Autodesk Inventor part; units mm, degrees
ref_plane "YZ Plane" through (0, 0, 0) normal (1, 0, 0) x (0, 1, 0)
ref_plane "XZ Plane" through (0, 0, 0) normal (0, 1, 0) x (-1, 0, 0)
ref_plane "XY Plane" through (0, 0, 0) normal (0, 0, 1) x (1, 0, 0)
sketch "Sketch1" plane through (0, 0, 0) normal (0, 1, 0) x (-1, 0, 0)
  line L0 (0, 0) -> (-21, 0) construction
  line L1 (-4.5, 4.5) -> (-16.5, 4.5)
  line L2 (-16.5, -4.5) -> (-4.5, -4.5)
  arc A0 (-4.5, -4.5) -> (-4.5, 4.5) centre (-4.5, 0) ccw
  arc A1 (-16.5, 4.5) -> (-16.5, -4.5) centre (-16.5, 0) ccw
  point P0 (-10.5, 0)
  dimension "d0" = 9
  dimension "d1" = 21
extrude "Extrusion1" add sketch "Sketch1" along normal blind 4
hole "Hole1" at (4.5, 4, 0) direction (0, -1, 0) diameter 4 end through all
hole "Hole2" at (16.5, 4, 0) direction (0, -1, 0) diameter 4 end through all
properties part number "A8-0015"
Verification items for the finished model (mm, model axes). Round coordinates to 2 decimals unless told otherwise and drop trailing zeros. Loops run counter-clockwise (first coordinate to the right, second up) from the corner with the lowest first, then second, coordinate; pieces in that order, holes last. Notation, with made-up numbers: (80.5, 73) - (89.5, 73) arc R14 cw to (89.5, 90) - close; hole circle Ø9 at (85.25, 33). An arc over 180 degrees is marked (long way). Use one line per item in the form item = value.
1. Section check D-D on z = -3.5. Record the cut outline in (x, y).
A:
outline = (1.67, 0) - (19.33, 0) - (19.33, 4) - (1.67, 4) - close
2. Scan lines: probe 1 along X at (y, z) = (1.15, 0); probe 2 along Z at (x, y) = (16.5, 1.9); probe 3 along Z at (x, y) = (18, 0.6). Record each from-to range of solid material in increasing order.
A:
probe_1 = 0 to 2.5, 6.5 to 14.5, 18.5 to 21
probe_2 = -4.5 to -2, 2 to 4.5
probe_3 = -4.24 to -1.32, 1.32 to 4.24
3. Section check B-B on x = 17.5. Record the cut outline in (y, z).
A:
outline = (0, -4.39) - (4, -4.39) - (4, -1.73) - (0, -1.73) - close; (0, 1.73) - (4, 1.73) - (4, 4.39) - (0, 4.39) - close
4. Gauge pin test, flat end, axial feed: pin 1 Ø1 at (y, z) = (2.5, -1) entering from -X. Record the tip position at first contact, or that the pin passes through.
A:
pin_1 = 0.03
5. Section check C-C on y = 2.95. Record the cut outline in (x, z).
A:
outline = (4.5, -4.5) - (16.5, -4.5) arc R4.5 ccw to (16.5, 4.5) - (4.5, 4.5) arc R4.5 ccw to start; hole circle Ø4 at (4.5, 0); hole circle Ø4 at (16.5, 0)
6. Draft check along X on faces 1 (the flat face through (10, 2, 4.5)), 2 (the cylindrical face through (21, 2, 0)), 3 (the cylindrical face through (6.452, 1.972, -0.434)). Enter one of: pulls with the +X half, pulls with the -X half, needs draft (parallel to the pull), parting line crosses it, or undercut.
A:
face_1 = needs draft
face_2 = pulls with the +X half
face_3 = undercut
7. Section check A-A on z = 0. Record the cut outline in (x, y).
A:
outline = (0, 0) - (2.5, 0) - (2.5, 4) - (0, 4) - close; (6.5, 0) - (14.5, 0) - (14.5, 4) - (6.5, 4) - close; (18.5, 0) - (21, 0) - (21, 4) - (18.5, 4) - close
